Can you work these out from the model? Positions are in its coordinate system, mm. A direction names the side the tool comes from. Give positions to 0.01 mm unless a question says otherwise; leave off trailing zeros. Order: outer loops, then holes, each group sorted by start corner. A loop starts at its lowest first (then second) coordinate and runs counter-clockwise, first axis right, second up. Notation, with made-up numbers: M 65.5,-0.5 L 110.5,-0.5 A8 cw 110.5,10.5 Z; hole C 69,79.5 d11. An arc over 180 degrees is marked long. Answer as a JSON object with one key per item and string values.
```python
from build123d import *

# Parameters (mm, degrees)
F0_W           = 60
F0_H           = 60
F1_DEPTH       = 3
F3_D           = 2.4384
F3_DEPTH       = 12.7
F3_CSINK_D     = 5.0038
F3_CSINK_ANGLE = 82
F3_TIP         = 0.7325692667
F4_R           = 5.08
F5_W           = 4
F5_H           = 49
F6_DEPTH       = 7
F7_R           = 2.54
F8_D           = 2.4384
F11_DEPTH      = 2


with BuildPart() as f1:
    # F0 (on Top) → F1 (new body)
    with BuildSketch(Plane.XY):
        Rectangle(F0_W, F0_H)
    extrude(amount=F1_DEPTH)

    # F3
    with Locations(Plane.XY.offset(3)):
        with Locations((-25, 25), (-25, -25), (25, -25), (25, 25)):
            CounterSinkHole(F3_D / 2, F3_CSINK_D / 2, depth=F3_DEPTH, counter_sink_angle=F3_CSINK_ANGLE)
            with Locations((0, 0, -(F3_DEPTH + F3_TIP / 2))):  # 118° drill point
                Cone(0, F3_D / 2, F3_TIP, mode=Mode.SUBTRACT)

    # F4
    f4_edges = [f1.edges().sort_by_distance(p)[0] for p in [
        (30, -30, 1.5),
        (-30, -30, 1.5),
        (30, 30, 1.5),
        (-30, 30, 1.5),
    ]]
    fillet(f4_edges, radius=F4_R)

    # F5 (on face) → F6 (join)
    with BuildSketch(Plane.XY.offset(3)):
        with Locations((32, 0)):
            Rectangle(F5_W, F5_H)
        with BuildLine():
            Line((30, -24.5), (30, 24.5))
            Line((30, 24.5), (27.4505423019, 24.5))
            ThreePointArc((27.4505423019, 24.5), (25, 22.498968698), (22.5494576981, 24.5))
            Line((22.5494576981, 24.5), (-22.5494576981, 24.5))
            ThreePointArc((-22.5494576981, 24.5), (-25, 22.498968698), (-27.4505423019, 24.5))
            Line((-27.4505423019, 24.5), (-30, 24.5))
            Line((-30, 24.5), (-30, -24.5))
            Line((-30, -24.5), (-27.4505423019, -24.5))
            ThreePointArc((-27.4505423019, -24.5), (-25, -22.498968698), (-22.5494576981, -24.5))
            Line((-22.5494576981, -24.5), (22.5494576981, -24.5))
            ThreePointArc((22.5494576981, -24.5), (25, -22.498968698), (27.4505423019, -24.5))
            Line((27.4505423019, -24.5), (30, -24.5))
        make_face()
        with Locations((-32, 0)):
            Rectangle(F5_W, F5_H)
    extrude(amount=F6_DEPTH)

    # F7
    f7_edges = [f1.edges().sort_by_distance(p)[0] for p in [
        (-34, -24.5, 6.5),
        (34, -24.5, 6.5),
        (34, 24.5, 6.5),
        (-34, 24.5, 6.5),
    ]]
    fillet(f7_edges, radius=F7_R)

    # F8 (through all)
    with Locations(Plane(origin=(0, 0, 0), x_dir=(1, 0, 0), z_dir=(0, 0, -1))):
        with Locations((0, 0)):
            Hole(F8_D / 2)

    # F10 (on face) → F11 (cut)
    with BuildSketch(Plane(origin=(0, 0, 0), x_dir=(1, 0, 0), z_dir=(0, 0, -1))):
        with BuildLine():
            Line((-0.9623644593, -1.3136032181), (-0.9623644593, -31.3395906546))
            Line((-0.9623644593, -31.3395906546), (1.0376355407, -31.3395906546))
            Line((1.0376355407, -31.3395906546), (1.0376355407, -1.2549945226))
            ThreePointArc((1.0376355407, -1.2549945226), (-0.0476988335, 1.6277050066), (-0.9623644593, -1.3136032181))
        make_face()
    extrude(amount=-F11_DEPTH, mode=Mode.SUBTRACT)


solid = f1.part
```
1) I want a section at D-D on y = 6. Write out the boundary of the cut face in (x, z), and give its area (3 significant figures).
Results found:
{"outline": "M -34,3 L -30,3 L -30,0 L -0.96,0 L -0.96,2 L 1.04,2 L 1.04,0 L 30,0 L 30,3 L 34,3 L 34,10 L -34,10 Z", "area": "652 mm²"}
2) I want a section at A-A on y = 0. Write out the boundary of the cut face in (x, z), and give its area (3 significant figures).
Results found:
{"outline": "M -34,3 L -30,3 L -30,0 L -1.63,0 L -1.63,2 L -1.22,2 L -1.22,10 L -34,10 Z; M 1.22,2 L 1.63,2 L 1.63,0 L 30,0 L 30,3 L 34,3 L 34,10 L 1.22,10 Z", "area": "630 mm²"}
3) I want a section at C-C on z = 3.75. Write out the boundary of the cut face in (x, y), and give its area (3 significant figures).
Results found:
{"outline": "M -34,-21.96 A2.54 ccw -31.46,-24.5 L -27.45,-24.5 A2.5 cw -22.55,-24.5 L 22.55,-24.5 A2.5 cw 27.45,-24.5 L 31.46,-24.5 A2.54 ccw 34,-21.96 L 34,21.96 A2.54 ccw 31.46,24.5 L 27.45,24.5 A2.5 cw 22.55,24.5 L -22.55,24.5 A2.5 cw -27.45,24.5 L -31.46,24.5 A2.54 ccw -34,21.96 Z; hole C 0,0 d2.44", "area": "3,290 mm²"}
4) I'm going to push flat-ended pins straight in: pin 1 Ø3 at (y, z) = (16, 2.5) entering from +X; pin 2 Ø1.5 at (x, z) = (13, 4.5) entering from +Y; pin 3 Ø3.5 at (y, z) = (-8.5, 1) entering from -X; pin 4 Ø3.5 at (x, z) = (-1.5, 5.5) entering from -Y. Where does each tip first touch, or does it pass through?
Results found:
{"pin 1": "stops at x = 34", "pin 2": "stops at y = 24.5", "pin 3": "stops at x = -30", "pin 4": "stops at y = -24.5"}
5) Thinking about a two-plate mould opening in Y: for faces 1 (the face through (-25, -22.5, 6.5)), 2 (the face through (25.26, 23.81, 0.75)), 3 (the face through (32, 0, 3)), 4 (the face through (33.276, 23.736, 6.549)), which applies, pulls with the +Y half, pulls with the -Y half, needs draft (parallel to the pull), parting line crosses it, or undercut?
Results found:
{"face 1": "pulls with the -Y half", "face 2": "undercut", "face 3": "needs draft", "face 4": "pulls with the +Y half"}
6) I need wall thicknesses on L1, parallel to Y at x = 25, z = 0.75; L2, parallel to X at y = 25, z = 1.15. Which ranges of each line are inside material? Lowest first, please.
Results found:
{"L1": "y = -30 to -26.22, -23.78 to 23.78, 26.22 to 30", "L2": "x = -30 to -26.22, -23.78 to -0.96, 1.04 to 23.78, 26.22 to 30"}
7) I want a section at B-B on x = 0. Write out the boundary of the cut face in (y, z).
Results found:
{"outline": "M -30,0 L -1.63,0 L -1.63,2 L -1.22,2 L -1.22,10 L -24.5,10 L -24.5,3 L -30,3 Z; M 1.22,2 L 30,2 L 30,3 L 24.5,3 L 24.5,10 L 1.22,10 Z"}
8) For faces 5 (the face through (29, 24.5, 6)), 6 (the face through (0, -24.5, 6)), 7 (the face through (-0.962, 15, 1)), which set-ups out of +Z, -Z, +X, -X, +Y, -Y let a thin tool reach every point of the face, with its end or its side?
Results found:
{"face 5": "+Z, +X, -X, +Y", "face 6": "+Z, +X, -X, -Y", "face 7": "-Z, +Y"}
